Read the model definition and answer for the solid it produces. Units are mm, in the model's axes. Face numbers are marked on the shaded views. A direction names the side the tool comes from. Give positions to 0.01 mm unless a question says otherwise; leave off trailing zeros. Write each loop counter-clockwise with the first axis right and the second up, starting at its lowest first coordinate (ties: lowest second). Pieces come first, ordered by that corner, then holes. Notation, with made-up numbers: M 84,21 L 117,21 A29 ccw 117,45 Z; hole C -34.5,68 d3. An arc over 180 degrees is marked long. Put each result on its own line as item: value.
from build123d import *

# Parameters (mm, degrees)
F1_DEPTH = 12.1
F2_T     = 1
F3_W     = 13.9636243694
F3_H     = 14.0063923318
F4_DEPTH = 25


with BuildPart() as f1:
    # F0 (on Top) → F1 (new body)
    with BuildSketch(Plane.XY):
        with BuildLine():
            Line((-4.25, 12.1212695545), (-3.5, 0))
            Line((-3.5, 0), (3.5, 0))
            Line((3.5, 0), (4.25, 12.1212695545))
            ThreePointArc((4.25, 12.1212695545), (0, 16), (-4.25, 12.1212695545))
        make_face()
    extrude(amount=F1_DEPTH)

    # F2
    f2_openings = [f1.faces().sort_by_distance(p)[0] for p in [
        (0, 7.847048, 12.1),
    ]]
    offset(amount=F2_T, openings=f2_openings, kind=Kind.INTERSECTION)

    # F3 (on face) → F4 (cut)
    with BuildSketch(Plane(origin=(0, 0, 0), x_dir=(-1, 0, 0), z_dir=(0, 1, 0))):
        with Locations((-0.2180829179, 5.7105472079)):
            Rectangle(F3_W, F3_H)
    extrude(amount=-F4_DEPTH, mode=Mode.SUBTRACT)


solid = f1.part
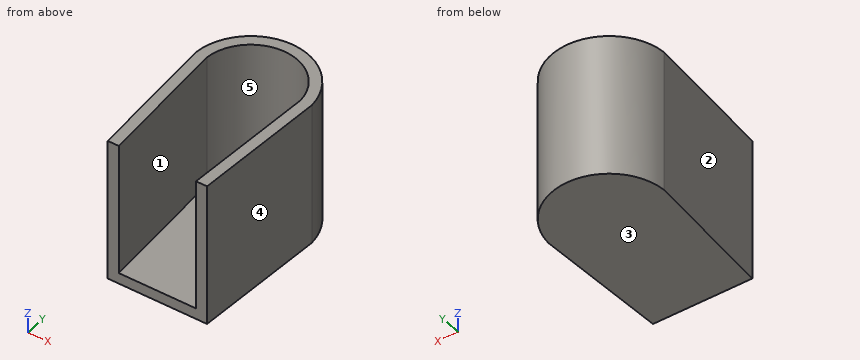
(1) Section D-D on x = 0.25 is taken. Determine the outline of the cut face in (y, z).
Result:
outline: M 0,-1 L 16.99,-1 L 16.99,12.1 L 15.99,12.1 L 15.99,0 L 0,0 Z
(2) Section B-B on y = 6.25 is taken. Determine the outline of the cut face in (x, z).
Result:
outline: M -4.89,-1 L 4.89,-1 L 4.89,12.1 L 3.89,12.1 L 3.89,0 L -3.89,0 L -3.89,12.1 L -4.89,12.1 Z
(3) Which of the six approach directions +Z, -Z, +X, -X, +Y, -Y give full straight-line access (tool end or side, diameter ignored) to the marked faces 1 and 2?
Result:
face 1: +Z
face 2: +Z, -Z, -X, -Y
(4) Section C-C on x = 2 is taken. Determine the outline of the cut face in (y, z), and give its area (3 significant figures).
Result:
outline: M 0,-1 L 16.61,-1 L 16.61,12.1 L 15.5,12.1 L 15.5,0 L 0,0 Z
area: 30.0 mm²
(5) Straight lines are drawn through the part: line 1 along Z through (x, y) = (-2, 2.75); line 2 along X through (y, z) = (2.25, 2.5); line 3 along X through (y, z) = (7.5, 1.5). For each, find the intervals that lie inside material, in ascending order. Write a range as from..to.
Result:
line 1: z = -1..0
line 2: x = -4.64..-3.64, 3.64..4.64
line 3: x = -4.97..-3.96, 3.96..4.97
(6) For a pull along Y with two mould halves and no side action, classify the marked faces 3, 4 and 5 as +Y half, -Y half, draft (parallel to the pull), parting line (faces both ways), or undercut.
Result:
face 3: draft
face 4: -Y half
face 5: undercut
(7) Given pin 1 Ø1.5 at (x, z) = (-4, 5.5) entering from +Y; pin 2 Ø1.5 at (y, z) = (6.5, 1.5) entering from +X; pin 3 Ø4 at (x, y) = (-1.5, 8) entering from +Z, each flat-ended and moving along its own axis, determine where each tip first touches the part or whether it passes through.
Result:
pin 1: stops at y = 15.88
pin 2: stops at x = 4.95
pin 3: stops at z = 0
(8) Section A-A on z = 1.75 is taken. Determine the outline of the cut face in (x, y), and give its area (3 significant figures).
Result:
outline: M -5.25,12.13 L -4.5,0 L -3.5,0 L -4.25,12.12 A4.27 cw 4.25,12.12 L 3.5,0 L 4.5,0 L 5.25,12.13 A5.27 ccw Z
area: 38.5 mm²
